Autodesk Inventor part; units mm, degrees
ref_plane "YZ Plane" through (0, 0, 0) normal (1, 0, 0) x (0, 1, 0)
ref_plane "XZ Plane" through (0, 0, 0) normal (0, 1, 0) x (-1, 0, 0)
ref_plane "XY Plane" through (0, 0, 0) normal (0, 0, 1) x (1, 0, 0)
sketch "Эскиз1" plane through (0, 0, 0) normal (0, 1, 0) x (-1, 0, 0)
  line L0 (0, 0) -> (-10, 0)
  line L1 (-10, 0) -> (-10, -18.8)
  line L2 (-10, -18.8) -> (0, -18.8)
  line L3 (0, -18.8) -> (0, 0)
  point P0 (0, 0)
  dimension "d0" = 10
  dimension "d1" = 18.8
extrude "Выдавливание1" add sketch "Эскиз1" along normal blind 7
sketch "Эскиз2" plane through (0, 7, 0) normal (0, 1, 0) x (1, 0, 0)
  line L0 (10, 0) -> (10, 18.8)
  line L1 (0, 0) -> (10, 0)
  line L2 (10, 0) -> (10, 10)
  line L3 (10, 10) -> (0, 10)
  line L4 (0, 10) -> (0, 0)
  dimension "d4" = 10
extrude "Выдавливание2" add sketch "Эскиз2" along normal blind 53
sketch "Эскиз4" plane through (0, 0, 0) normal (0, -1, 0) x (1, 0, 0)
  line L0 (0, 0) -> (10, 0)
  line L1 (0, 0) -> (10, 0)
  line L2 (10, 0) -> (10, -10)
  line L3 (10, -10) -> (0, -10)
  line L4 (0, -10) -> (0, 0)
  line L5 (0, -10) -> (10, -10)
  line L6 (10, -10) -> (10, -18.8)
  line L7 (10, -18.8) -> (0, -18.8)
  line L8 (0, -18.8) -> (0, -10)
  point P0 (5, -5)
  point P1 (5, -14.4)
  point P2 (5, 0)
  point P3 (10, -5)
  point P4 (10, -14.4)
hole "Отверстие1" at (5, 0, -5) at (5, 0, -14.4) direction (0, 1, 0) diameter 2.8 depth 7
sketch "Эскиз7" plane through (0, 0, 0) normal (0, 0, 1) x (1, 0, 0)
  line L0 (0, 0) -> (10, 0)
  line L1 (0, 60) -> (10, 60)
  point P0 (5, 10)
  point P1 (5, 50)
  point P2 (5, 0)
  dimension "d21" = 10
  dimension "d22" = 10
hole "Отверстие2" at (5, 10, 0) at (5, 50, 0) direction (0, 0, -1) diameter 2.8 end through all
sketch "Эскиз9" plane through (0, 60, 0) normal (0, 1, 0) x (1, 0, 0)
  circle A0 centre (5, 5) radius 1.4
  point P0 (0, 0)
hole "Отверстие3" at (5, 60, -5) direction (0, -1, 0) diameter 2.8 depth 7
sketch "Эскиз11" plane through (0, 0, -18.8) normal (-1, 0, 0) x (0, 0, 1)
  line L0 (8.8, 60) -> (18.8, 60)
  line L1 (0, 0) -> (18.8, 0)
  point P0 (13.8, 14)
  point P1 (13.8, 46)
  point P2 (13.8, 60)
  dimension "d37" = 14
  dimension "d38" = 14
hole "Отверстие4" at (0, 14, -5) at (0, 46, -5) direction (1, 0, 0) diameter 2.8 end through all
properties part number "StructureCenter"
Source: CAD feature listing. Evaluate the final solid. Frame: model axes, mm. A direction names the side the tool comes from. Coordinates: 2 decimals unless noted, no trailing zeros. Write each loop counter-clockwise with the first axis right and the second up, starting at its lowest first coordinate (ties: lowest second). Pieces come first, ordered by that corner, then holes. Notation, with made-up numbers: (55, 18.25) -> (81, 18.25) arc R27 ccw to (81, 51.25) -> close; hole circle Ø6 at (65.25, 5.25). An arc over 180 degrees is marked (long way). Return JSON: item names as keys, results as strings. Group by question number.
1) Section query A-A, the plane z = -14.4. Return loops of the section in (x, y), plus the area to 3 significant figures.
2) Contact query for flat-ended pins moving along their axis: P1, Ø2.5, axis at x = 5, y = 10, coming from the -Z side; P2, Ø2.5, axis at x = 5, z = -5, coming from the -Y side; P3, Ø3.5, axis at x = 5, z = -14.4, coming from the +Y side; P4, Ø1.5, axis at x = 3, y = 21, coming from the -Z side. Output: stop coordinate, or through.
3) Mould query, pull axis Z, two halves, no side actions, for faces 1 (the face through (5, 7, -5)), 2 (the face through (6, 7, -13)), 3 (the face through (5, 3, -18.8)). Classes: +Z half, -Z half, draft (parallel to the pull), parting line (faces both ways), or undercut.
4) Section query C-C, the plane x = 5. Return loops of the section in (y, z).
5) Section query D-D, the plane x = 9.25. Return loops of the section in (y, z), plus the area to 3 significant figures.
6) Set-up query: faces 4 (the face through (5.54, 56.45, -3.71)), 5 (the face through (5, 30, 0)), 6 (the face through (5.54, 3.55, -6.29)), 7 (the face through (5, 33, -10)). Return all of +Z, -Z, +X, -X, +Y, -Y with unobstructed straight access to the full face (end or side cutting, diameter ignored); none if empty.
7) Section query B-B, the plane y = 14. Return loops of the section in (x, z), plus the area to 3 significant figures.
8) Ray query, line 1 along Y through (x, z) = (5, -2); line 2 along Z through (x, y) = (4.25, 46); line 3 along X through (y, z) = (10, -3.75). Return the intervals inside material, ascending.
From the geometry:
{
 "1": {"outline": "(0, 0) -> (3.6, 0) -> (3.6, 7) -> (0, 7) -> close; (6.4, 0) -> (10, 0) -> (10, 7) -> (6.4, 7) -> close", "area": "50.4 mm²"},
 "2": {"P1": "through", "P2": "y = 7", "P3": "y = 7", "P4": "z = -10"},
 "3": {"face 1": "undercut", "face 2": "draft", "face 3": "-Z half"},
 "4": {"outline": "(0, -18.8) -> (7, -18.8) -> (7, -15.8) -> (0, -15.8) -> close; (0, -13) -> (7, -13) -> (7, -10) -> (8.6, -10) -> (8.6, 0) -> (0, 0) -> (0, -3.6) -> (7, -3.6) -> (7, -6.4) -> (0, -6.4) -> close; (11.4, -10) -> (48.6, -10) -> (48.6, 0) -> (11.4, 0) -> close; (51.4, -10) -> (60, -10) -> (60, -6.4) -> (53, -6.4) -> (53, -3.6) -> (60, -3.6) -> (60, 0) -> (51.4, 0) -> close; hole circle Ø2.8 at (14, -5); hole circle Ø2.8 at (46, -5)"},
 "5": {"outline": "(0, -18.8) -> (7, -18.8) -> (7, -10) -> (60, -10) -> (60, 0) -> (0, 0) -> close; hole circle Ø2.8 at (14, -5); hole circle Ø2.8 at (46, -5)", "area": "649 mm²"},
 "6": {"face 4": "+Y", "face 5": "+Z, +X, -X, +Y, -Y", "face 6": "-Y", "face 7": "-Z, +X, -X, +Y"},
 "7": {"outline": "(0, -10) -> (10, -10) -> (10, -6.4) -> (0, -6.4) -> close; (0, -3.6) -> (10, -3.6) -> (10, 0) -> (0, 0) -> close", "area": "72.0 mm²"},
 "8": {"line 1": "0 to 8.6, 11.4 to 48.6, 51.4 to 60", "line 2": "-10 to -6.4, -3.6 to 0", "line 3": "0 to 3.6, 6.4 to 10"}
}
